Geometry check sheet. Reference: the model listing, model coordinates, mm. Face numbers are marked on the shaded views. Round coordinates to 2 decimals unless told otherwise and drop trailing zeros. Use a Markdown table: item, result. Add a question column.
Q1. Sectioned sample at A-A, the plane y = 163.5. Give the number of separate pieces and of enclosed holes in the cut face, then the cut area to 3 significant figures.
Q2. Material ranges on L1, parallel to Z at x = 44.75, y = 111.5; L2, parallel to Z at x = 25, y = 166; L3, parallel to Z at x = 17.5, y = 156.5, recorded low to high.
Q3. Release check for a two-part mould opening along X. For the marked faces 1, 2, 3 and 4 record: released by +X, released by -X, zero draft, split by the parting line, or undercut.
Q4. Gauge pin test, flat ends, axial feed: P1, Ø6, axis at x = 50.5, y = 50, coming from the -Z side; P2, Ø8, axis at y = 155.5, z = 88.5, coming from the +X side; P3, Ø2, axis at x = 44.5, y = 20, coming from the +Z side. Record the tip position at first contact, or that the pin passes through.
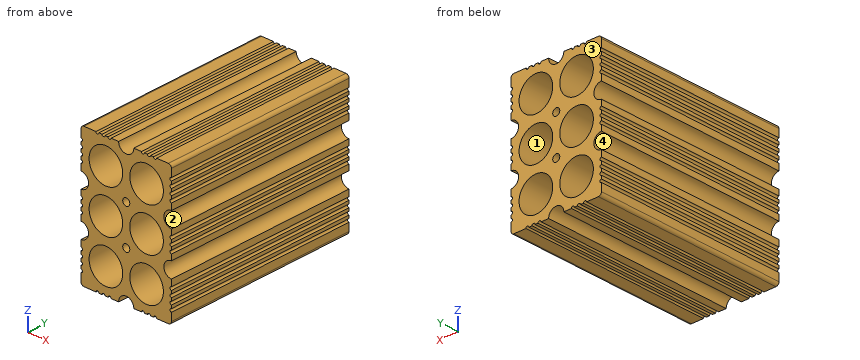
Autodesk Inventor part; units mm, degrees
ref_plane "YZ Plane" through (0, 0, 0) normal (1, 0, 0) x (0, 1, 0)
ref_plane "XZ Plane" through (0, 0, 0) normal (0, 1, 0) x (-1, 0, 0)
ref_plane "XY Plane" through (0, 0, 0) normal (0, 0, 1) x (1, 0, 0)
sketch "Sketch1" plane through (0, 0, 0) normal (0, 0, 1) x (1, 0, 0)
  line L0 (0, 0) -> (89.5, 0)
  line L1 (89.5, 0) -> (89.5, 188.8)
  line L2 (89.5, 188.8) -> (0, 188.8)
  line L3 (0, 188.8) -> (0, 0)
  dimension "d0" = 89.5
  dimension "d1" = 188.8
extrude "Corpo" add sketch "Sketch1" along normal blind 131.8
sketch "Furações" plane through (0, 0, 0) normal (0, -1, 0) x (1, 0, 0)
  line L0 (89.5, 131.8) -> (0, 131.8)
  line L1 (89.5, 0) -> (0, 0)
  line L2 (44.75, 131.8) -> (44.75, 84.8) construction
  line L3 (44.75, 0) -> (44.75, 47) construction
  circle A0 centre (44.75, 84.8) radius 3.5
  circle A1 centre (44.75, 47) radius 3.5
  line L4 (89.5, 123.8) -> (0, 123.8) construction
  line L5 (8, 0) -> (8, 131.8) construction
  line L6 (41.25, 131.8) -> (41.25, 84.8) construction
  circle A2 centre (24.625, 107.175) radius 16.625
  line L7 (0, 0) -> (0, 131.8) construction
  line L8 (0, 65.9) -> (89.5, 65.9) construction
  line L9 (89.5, 0) -> (89.5, 131.8)
  line L10 (24.625, 131.8) -> (156.425, 131.8) construction
  circle A3 centre (24.625, 65.9) radius 16.625
  line L11 (0, 8) -> (89.5, 8) construction
  line L12 (41.25, 0) -> (41.25, 47) construction
  circle A4 centre (24.625, 24.625) radius 16.625
  circle A5 centre (64.875, 107.175) radius 16.625
  circle A6 centre (64.875, 65.9) radius 16.625
  circle A7 centre (64.875, 24.625) radius 16.625
  circle A8 centre (44.75, 131.8) radius 7.5
  circle A9 centre (44.75, 0) radius 7.5
  line L13 (24.625, 131.8) -> (24.625, 123.8) construction
  line L14 (24.625, 90.55) -> (24.625, 82.525) construction
  line L15 (24.625, 49.275) -> (24.625, 41.25) construction
  line L16 (24.625, 8) -> (24.625, 0) construction
  line L17 (24.625, 86.5375) -> (0, 86.5375) construction
  line L18 (24.625, 45.2625) -> (0, 45.2625) construction
  circle A10 centre (0, 86.5375) radius 7.5
  circle A11 centre (0, 45.2625) radius 7.5
  circle A12 centre (89.5, 86.5375) radius 7.5
  circle A13 centre (89.5, 45.2625) radius 7.5
  line L19 (0, 123.8) -> (0, 119.8) construction
  circle A14 centre (0, 119.8) radius 1.5
  line L20 (0, 119.8) -> (0, 113.8) construction
  circle A15 centre (0, 113.8) radius 1.5
  line L21 (0, 113.8) -> (0, 107.8) construction
  circle A16 centre (0, 107.8) radius 1.5
  line L22 (0, 107.8) -> (0, 101.8) construction
  circle A17 centre (0, 101.8) radius 1.5
  circle A18 centre (0, 65.9) radius 1.5
  line L23 (0, 65.9) -> (0, 71.9) construction
  line L24 (0, 65.9) -> (0, 59.9) construction
  circle A19 centre (0, 71.9) radius 1.5
  circle A20 centre (0, 59.9) radius 1.5
  line L25 (0, 8) -> (0, 12) construction
  circle A21 centre (0, 12) radius 1.5
  line L26 (0, 12) -> (0, 18) construction
  circle A22 centre (0, 18) radius 1.5
  line L27 (0, 18) -> (0, 24) construction
  circle A23 centre (0, 24) radius 1.5
  line L28 (0, 24) -> (0, 30) construction
  circle A24 centre (0, 30) radius 1.5
  line L29 (37.25, 0) -> (28.25, 0) construction
  circle A25 centre (28.25, 0) radius 1.5
  line L30 (28.25, 0) -> (22.25, 0) construction
  circle A26 centre (22.25, 0) radius 1.5
  line L31 (22.25, 0) -> (16.25, 0) construction
  circle A27 centre (16.25, 0) radius 1.5
  circle A28 centre (28.25, 131.8) radius 1.5
  line L32 (28.25, 131.8) -> (22.25, 131.8) construction
  circle A29 centre (22.25, 131.8) radius 1.5
  line L33 (22.25, 131.8) -> (16.25, 131.8) construction
  circle A30 centre (16.25, 131.8) radius 1.5
  circle A31 centre (89.5, 119.8) radius 1.5
  circle A32 centre (89.5, 113.8) radius 1.5
  circle A33 centre (89.5, 107.8) radius 1.5
  circle A34 centre (89.5, 101.8) radius 1.5
  circle A35 centre (89.5, 65.9) radius 1.5
  circle A36 centre (89.5, 71.9) radius 1.5
  circle A37 centre (89.5, 59.9) radius 1.5
  circle A38 centre (89.5, 12) radius 1.5
  circle A39 centre (89.5, 18) radius 1.5
  circle A40 centre (89.5, 24) radius 1.5
  circle A41 centre (89.5, 30) radius 1.5
  circle A42 centre (61.25, 0) radius 1.5
  circle A43 centre (67.25, 0) radius 1.5
  circle A44 centre (73.25, 0) radius 1.5
  circle A45 centre (73.25, 131.8) radius 1.5
  circle A46 centre (67.25, 131.8) radius 1.5
  circle A47 centre (61.25, 131.8) radius 1.5
  dimension "d4" = 47
  dimension "d5" = 47
  dimension "d6" = 7
  dimension "d7" = 7
  dimension "d8" = 8
  dimension "d9" = 8
  dimension "d10" = 3.5
  dimension "d12" = 33.25
  dimension "d13" = 3.5
  dimension "d14" = 15
  dimension "d15" = 15
  dimension "d16" = 15
  dimension "d17" = 4
  dimension "d18" = 3
  dimension "d19" = 6
  dimension "d20" = 3
  dimension "d21" = 6
  dimension "d22" = 3
  dimension "d23" = 6
  dimension "d24" = 3
  dimension "d25" = 3
  dimension "d26" = 6
  dimension "d27" = 6
  dimension "d28" = 3
  dimension "d29" = 3
  dimension "d30" = 4
  dimension "d31" = 3
  dimension "d32" = 6
  dimension "d33" = 3
  dimension "d34" = 6
  dimension "d35" = 3
  dimension "d36" = 6
  dimension "d37" = 3
  dimension "d38" = 9
  dimension "d39" = 3
  dimension "d40" = 6
  dimension "d41" = 3
  dimension "d42" = 6
  dimension "d43" = 3
extrude "furação" cut sketch "Furações" against normal up to surface (188.8 mm away)
fillet "Fillet1" radius 3 4 edges at (0, 94.4, 131.8) (89.5, 94.4, 131.8) (89.5, 94.4, 0) (0, 94.4, 0)
properties part number "Tijolo 9x19cm" material "Gold"
Values:
| question | item | result |
|---|---|---|
| 1 | separate pieces | 1 |
| 1 | enclosed holes | 8 |
| 1 | area | 5,850 mm^2 |
| 2 | L1 | 7.5 to 43.5, 50.5 to 81.3, 88.3 to 124.3 |
| 2 | L2 | 0 to 8, 41.25 to 49.28, 82.52 to 90.55, 123.8 to 131.8 |
| 2 | L3 | 0.83 to 9.6, 39.65 to 50.88, 80.92 to 92.15, 122.2 to 130.97 |
| 3 | face 1 | undercut |
| 3 | face 2 | released by +X |
| 3 | face 3 | zero draft |
| 3 | face 4 | released by -X |
| 4 | P1 | z = 0 |
| 4 | P2 | x = 84.95 |
| 4 | P3 | z = 124.4 |
